from build123d import *

# Parameters (mm, degrees)
BOSS_EXTRUDE1_DEPTH = 5
SKETCH2_R           = 1.95
SKETCH2_W           = 22
SKETCH2_H           = 23
CUT_EXTRUDE1_DEPTH  = 6


with BuildPart() as part:
    # Sketch1 → Boss-Extrude1 (new body)
    with BuildSketch(Plane(origin=(0, 0, 0), x_dir=(1, 0, 0), z_dir=(0, 1, 0))):
        with BuildLine():
            Line((-36, 0), (-2, 0))
            ThreePointArc((-2, 0), (-0.585786438, -0.585786438), (0, -2))
            Line((0, -2), (0, -47.22))
            ThreePointArc((0, -47.22), (-0.585786438, -48.634213562), (-2, -49.22))
            Line((-2, -49.22), (-36, -49.22))
            ThreePointArc((-36, -49.22), (-37.414213562, -48.634213562), (-38, -47.22))
            Line((-38, -47.22), (-38, -2))
            ThreePointArc((-38, -2), (-37.414213562, -0.585786438), (-36, 0))
        make_face()
    extrude(amount=BOSS_EXTRUDE1_DEPTH)

    # Sketch2 → Cut-Extrude1 (cut, through all)
    with BuildSketch(Plane(origin=(0, 5, 0), x_dir=(1, 0, 0), z_dir=(0, 1, 0))):
        with Locations((-4, -4)):
            Circle(SKETCH2_R)
        with Locations((-14, -4)):
            Circle(SKETCH2_R)
        with Locations((-24, -4)):
            Circle(SKETCH2_R)
        with Locations((-54, -4)):
            Circle(SKETCH2_R)
        with Locations((-34, -4)):
            Circle(SKETCH2_R)
        with Locations((-44, -4)):
            Circle(SKETCH2_R)
        with Locations((-44, -45.22)):
            Circle(SKETCH2_R)
        with Locations((-34, -45.22)):
            Circle(SKETCH2_R)
        with Locations((-54, -45.22)):
            Circle(SKETCH2_R)
        with Locations((-24, -45.22)):
            Circle(SKETCH2_R)
        with Locations((-14, -45.22)):
            Circle(SKETCH2_R)
        with Locations((-4, -45.22)):
            Circle(SKETCH2_R)
        with Locations((-19, -24.61)):
            Rectangle(SKETCH2_W, SKETCH2_H)
    extrude(amount=-CUT_EXTRUDE1_DEPTH, mode=Mode.SUBTRACT)


solid = part.part
Model file for the job. Use its own axes, mm. A direction names the side the tool comes from. Give positions to 0.01 mm unless a question says otherwise; leave off trailing zeros. Loops run counter-clockwise (first coordinate to the right, second up) from the corner with the lowest first, then second, coordinate; pieces in that order, holes last.
Item 1: Which spindle directions (+Z, -Z, +X, -X, +Y, -Y) get a long thin tool onto all of the face, cutting with end or side? Do faces 1 (the face through (-19, 3, 36.11)), 2 (the face through (-0.6, 2.46, 0.57)). Say none if no direction does.
Check values:
face 1: +Y, -Y
face 2: -Z, +X, +Y, -Y
Item 2: Slice it at A-A (x = -29). Write the cut outline in (y, z).
Check values:
outline: (0, 0) - (5, 0) - (5, 13.11) - (0, 13.11) - close; (0, 36.11) - (5, 36.11) - (5, 49.22) - (0, 49.22) - close
Item 3: Slice it at D-D (x = -14). Write the cut outline in (y, z), plus the area to 3 significant figures.
Check values:
outline: (0, 0) - (5, 0) - (5, 2.05) - (0, 2.05) - close; (0, 5.95) - (5, 5.95) - (5, 13.11) - (0, 13.11) - close; (0, 36.11) - (5, 36.11) - (5, 43.27) - (0, 43.27) - close; (0, 47.17) - (5, 47.17) - (5, 49.22) - (0, 49.22) - close
area: 92.1 mm2
Item 4: Drop a flat-ended pin along its axis: P1, Ø3, axis at x = -14, z = 4, coming from the +Y side. Give the stop position or say it passes through.
Check values:
P1: passes through
Item 5: Slice it at B-B (z = 4). Write the cut outline in (x, y), plus the area to 3 significant figures.
Check values:
outline: (-38, 0) - (-35.95, 0) - (-35.95, 5) - (-38, 5) - close; (-32.05, 0) - (-25.95, 0) - (-25.95, 5) - (-32.05, 5) - close; (-22.05, 0) - (-15.95, 0) - (-15.95, 5) - (-22.05, 5) - close; (-12.05, 0) - (-5.95, 0) - (-5.95, 5) - (-12.05, 5) - close; (-2.05, 0) - (0, 0) - (0, 5) - (-2.05, 5) - close
area: 112 mm2
Item 6: Mould opens along X. For faces 3 (the face through (-24.423, 2.535, 47.124)), 4 (the face through (-33.1, 2.54, 46.95)), 5 (the face through (-0.57, 2.46, 48.62)), 6 (the face through (-37.43, 2.46, 0.6)) say: +X half, -X half, draft (parallel to the pull), parting line (faces both ways), or undercut.
Check values:
face 3: undercut
face 4: undercut
face 5: +X half
face 6: -X half
Item 7: Slice it at C-C (y = 3.5). Give the number of separate pieces and of enclosed holes in the cut face, plus the area to 3 significant figures.
Check values:
separate pieces: 1
enclosed holes: 9
area: 1,270 mm2
Item 8: Drill centre lines: line 1 along Z through (x, y) = (-24, 2.9); line 2 along X through (y, z) = (1.95, 4); line 3 along Z through (x, y) = (-4, 1.15). Where is each one in solid material? Low to high.
Check values:
line 1: z = 0 to 2.05, 5.95 to 13.11, 36.11 to 43.27, 47.17 to 49.22
line 2: x = -38 to -35.95, -32.05 to -25.95, -22.05 to -15.95, -12.05 to -5.95, -2.05 to 0
line 3: z = 0 to 2.05, 5.95 to 43.27, 47.17 to 49.22
